Read the model definition and answer for the solid it produces. Units are mm, in the model's axes. A direction names the side the tool comes from. Give positions to 0.01 mm unless a question says otherwise; leave off trailing zeros. Loops run counter-clockwise (first coordinate to the right, second up) from the corner with the lowest first, then second, coordinate; pieces in that order, holes last. Notation, with made-up numbers: (-23.5, 42) - (-16.5, 42) arc R22 cw to (-16.5, 79) - close; hole circle Ø9 at (20.5, 39). An arc over 180 degrees is marked (long way). Put each result on its own line as item: value. Start each with the question number.
1. Consider L1, parallel to Y at x = -35, z = -5.5; L2, parallel to Z at x = 20, y = 30; L3, parallel to Z at x = 12, y = 13. Determine where each line is inside the solid, lowest interval first. Write a range as from..to.
2. For a pull along Y with two mould halves and no side action, classify faces 5 (the cylindrical face through (-4.487, 6.989, -9.318)), 6 (the flat face through (-48.834, 35, -9)), 7 (the cylindrical face through (20.45, 50.453, -16.416)), 8 (the cylindrical face through (20.45, 50.453, 18.063)) as released by +Y, released by -Y, zero draft, split by the parting line, or undercut.
3. A cutting plane is placed at C-C, the plane y = 30. Determine the outline of the cut face in (x, z).
4. A cutting plane is placed at A-A, the plane z = 15.5. Determine the outline of the cut face in (x, y).
5. For faces 1 (the flat face through (-38, 51, -9)), 2 (the flat face through (-24.641, 49.203, -9.685)), 3 (the flat face through (16, 41, 13.5)), 4 (the flat face through (-16.834, 34, 13)), determine the directions among +Z, -Z, +X, -X, +Y, -Y from which every point of the face is accessible in a straight line to the end or side of a thin tool.
6. Given pin 1 Ø7.5 at (x, z) = (-38.5, -11.5) entering from +Y; pin 2 Ø2 at (y, z) = (20.5, 12.5) entering from +X; pin 3 Ø2 at (x, z) = (-21, -3) entering from -Y, each flat-ended and moving along its own axis, determine where each tip first touches the part or whether it passes through.
7. A cutting plane is placed at D-D, the plane y = 45. Determine the outline of the cut face in (x, z), plus the area to 3 significant figures.
8. A cutting plane is placed at B-B, the plane z = -17.5. Determine the outline of the cut face in (x, y), plus the area to 3 significant figures.
```python
from build123d import *

# Parameters (mm, degrees)
BOSS_EXTRU_1_DEPTH      = 22.5
ESQUISSE2_R             = 7
ENL_V_MAT_EXTRU_1_DEPTH = 89.82992258
ENL_V_MAT_EXTRU_2_DEPTH = 19
ENL_V_START             = -9
ENL_V_MAT_EXTRU_3_DEPTH = 24
ESQUISSE6_R             = 5.5
ENL_V_MAT_EXTRU_4_DEPTH = 89.82992258


with BuildPart() as part:
    # Esquisse1 → Boss.-Extru.1 (new, symmetric)
    with BuildSketch(Plane.XY):
        with BuildLine():
            Line((0, 0), (6.166045157, 0))
            Line((6.166045157, 0), (35.166045157, 35))
            Line((35.166045157, 35), (35.166045157, 54))
            Line((35.166045157, 54), (30.166045157, 59))
            Line((30.166045157, 59), (6.166045157, 59))
            ThreePointArc((6.166045157, 59), (-2.242317514, 49.535902458), (-14.729912491, 47.455114912))
            Line((-14.729912491, 47.455114912), (-34.833954843, 51))
            Line((-34.833954843, 51), (-41.833954843, 51))
            Line((-41.833954843, 51), (-48.833954843, 44))
            Line((-48.833954843, 44), (-48.833954843, 26))
            Line((-48.833954843, 26), (-41.833954843, 19))
            Line((-41.833954843, 19), (-11.721441141, 19))
            ThreePointArc((-11.721441141, 19), (-8.45620536, 17.786586232), (-6.7758024, 14.735294118))
            ThreePointArc((-6.7758024, 14.735294118), (-4.438972197, 6.884327939), (0, 0))
        make_face()
    extrude(amount=BOSS_EXTRU_1_DEPTH, both=True)

    # Esquisse2 → Enlèv. mat.-Extru.1 (cut, through all)
    with BuildSketch(Plane.XY.offset(22.5)):
        with Locations((-34.833954843, 33)):
            Circle(ESQUISSE2_R)
    extrude(amount=-ENL_V_MAT_EXTRU_1_DEPTH, mode=Mode.SUBTRACT)

    # Esquisse4 → Enlèv. mat.-Extru.2 (cut)
    with BuildSketch(Plane.XY.offset(22.5)):
        Polygon((-16.833954843, 47.826114347), (-16.833954843, 19), (-41.833954843, 19), (-48.833954843, 26), (-48.833954843, 44), (-41.833954843, 51), (-34.833954843, 51), align=None)
        with BuildLine():
            Line((-11.721441141, 19), (21.9089023, 19))
            Line((21.9089023, 19), (6.166045157, 0))
            Line((6.166045157, 0), (0, 0))
            ThreePointArc((0, 0), (-4.438972197, 6.884327939), (-6.7758024, 14.735294118))
            ThreePointArc((-6.7758024, 14.735294118), (-8.45620536, 17.786586232), (-11.721441141, 19))
        make_face()
    extrude(amount=-ENL_V_MAT_EXTRU_2_DEPTH, mode=Mode.SUBTRACT)

    # Esquisse5 → Enlèv. mat.-Extru.3 (cut)
    with BuildSketch(Plane.XY.offset(22.5).offset(ENL_V_START)):
        with BuildLine():
            Line((25.223188014, 23), (35.166045157, 35))
            Line((35.166045157, 35), (35.166045157, 54))
            Line((35.166045157, 54), (30.166045157, 59))
            Line((30.166045157, 59), (6.166045157, 59))
            ThreePointArc((6.166045157, 59), (2.323444718, 53.058207825), (-3.426832653, 48.93452227))
            ThreePointArc((-3.426832653, 48.93452227), (7.650971958, 32.380053701), (25.223188014, 23))
        make_face()
    extrude(amount=-ENL_V_MAT_EXTRU_3_DEPTH, mode=Mode.SUBTRACT)

    # Esquisse6 → Enlèv. mat.-Extru.4 (cut, through all)
    with BuildSketch(Plane.XY.offset(22.5)):
        with Locations((21.166045157, 45)):
            Circle(ESQUISSE6_R)
    extrude(amount=-ENL_V_MAT_EXTRU_4_DEPTH, mode=Mode.SUBTRACT)


solid = part.part
```
Return value:
1. L1: y = 19..26, 40..51
1. L2: z = -22.5..-10.5, 13.5..22.5
1. L3: z = -22.5..3.5
2. face 5: released by -Y
2. face 6: zero draft
2. face 7: undercut
2. face 8: undercut
3. outline: (-48.83, -22.5) - (-41.16, -22.5) - (-41.16, 3.5) - (-48.83, 3.5) - close; (-28.51, -22.5) - (31.02, -22.5) - (31.02, -10.5) - (10.53, -10.5) - (10.53, 13.5) - (31.02, 13.5) - (31.02, 22.5) - (-16.83, 22.5) - (-16.83, 3.5) - (-28.51, 3.5) - close
4. outline: (-16.83, 19) - (21.91, 19) - (35.17, 35) - (35.17, 54) - (30.17, 59) - (6.17, 59) arc R19 cw to (-14.73, 47.46) - (-16.83, 47.83) - close; hole circle Ø11 at (21.17, 45)
5. face 1: +Z, -Z, -X, +Y
5. face 2: +Z, -Z, +Y
5. face 3: +X, +Y
5. face 4: +Z, -X, +Y, -Y
6. pin 1: stops at y = 51
6. pin 2: stops at x = 23.98
6. pin 3: stops at y = 19
7. outline: (-47.83, -22.5) - (15.67, -22.5) - (15.67, -10.5) - (-1.78, -10.5) - (-1.78, 13.5) - (15.67, 13.5) - (15.67, 22.5) - (-16.83, 22.5) - (-16.83, 3.5) - (-47.83, 3.5) - close; (26.67, -22.5) - (35.17, -22.5) - (35.17, -10.5) - (26.67, -10.5) - close; (26.67, 13.5) - (35.17, 13.5) - (35.17, 22.5) - (26.67, 22.5) - close
7. area: 2,030 mm2
8. outline: (-48.83, 26) - (-41.83, 19) - (-11.72, 19) arc R5 cw to (-6.78, 14.74) arc R29 ccw to (0, 0) - (6.17, 0) - (35.17, 35) - (35.17, 54) - (30.17, 59) - (6.17, 59) arc R19 cw to (-14.73, 47.46) - (-34.83, 51) - (-41.83, 51) - (-48.83, 44) - close; hole circle Ø14 at (-34.83, 33); hole circle Ø11 at (21.17, 45)
8. area: 2,810 mm2
